Design review of the part built by this model. Coordinates are the model's own, in mm. Face numbers are marked on the shaded views. A direction names the side the tool comes from. Coordinates: 2 decimals unless noted, no trailing zeros. Write each loop counter-clockwise with the first axis right and the second up, starting at its lowest first coordinate (ties: lowest second). Pieces come first, ordered by that corner, then holes. Notation, with made-up numbers: (-19.5, 29.5) - (22.5, 29.5) arc R26 cw to (22.5, 52.5) - close; hole circle Ø3 at (89, 16). An arc over 180 degrees is marked (long way). Answer as a JSON object with one key per item and string values.
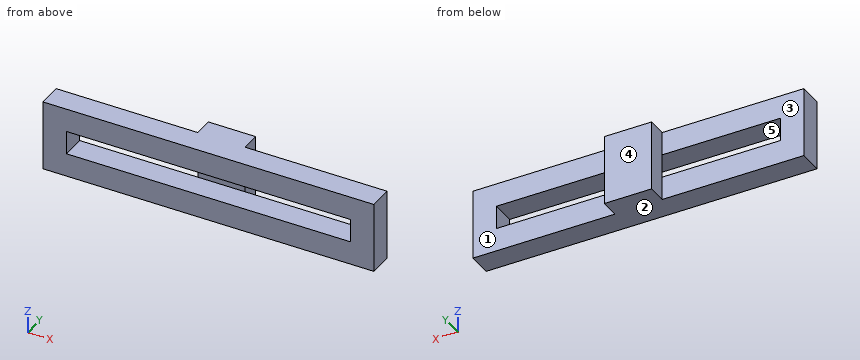
```python
from build123d import *

# Parameters (mm, degrees)
SKETCH2_W           = 70
SKETCH2_H           = 15
SKETCH2_W_2         = 60
SKETCH2_H_2         = 5
BOSS_EXTRUDE3_DEPTH = 5
SKETCH3_W           = 10
SKETCH3_H           = 15
BOSS_EXTRUDE4_DEPTH = 4


with BuildPart() as part:
    # Sketch2 → Boss-Extrude3 (new body)
    with BuildSketch(Plane(origin=(0, 0, 0), x_dir=(1, 0, 0), z_dir=(0, 1, 0))):
        Rectangle(SKETCH2_W, SKETCH2_H)
        Rectangle(SKETCH2_W_2, SKETCH2_H_2, mode=Mode.SUBTRACT)
    extrude(amount=BOSS_EXTRUDE3_DEPTH)

    # Sketch3 → Boss-Extrude4 (add)
    with BuildSketch(Plane(origin=(0, 5, 0), x_dir=(1, 0, 0), z_dir=(0, 1, 0))):
        Rectangle(SKETCH3_W, SKETCH3_H)
    extrude(amount=BOSS_EXTRUDE4_DEPTH)


solid = part.part
```
(1) Take a section at B-B, the plane y = 3.25. Write out the cut boundary in (x, z).
Solved:
{"outline": "(-35, -7.5) - (35, -7.5) - (35, 7.5) - (-35, 7.5) - close; hole (-30, -2.5) - (30, -2.5) - (30, 2.5) - (-30, 2.5) - close"}
(2) Take a section at D-D, the plane z = 6.75. Write out the cut boundary in (x, y).
Solved:
{"outline": "(-35, 0) - (35, 0) - (35, 5) - (5, 5) - (5, 9) - (-5, 9) - (-5, 5) - (-35, 5) - close"}
(3) Take a section at C-C, the plane x = 14. Write out the cut boundary in (y, z), and give its area (3 significant figures).
Solved:
{"outline": "(0, -7.5) - (5, -7.5) - (5, -2.5) - (0, -2.5) - close; (0, 2.5) - (5, 2.5) - (5, 7.5) - (0, 7.5) - close", "area": "50.0 mm^2"}
(4) For pin 1 (3 mm diameter, centred on y = 7, z = -3.5, fed in from +X); pin 2 (4.5 mm diameter, centred on x = 19.5, z = 2.5, fed in from +Y); pin 3 (4.5 mm diameter, centred on y = 7.5, z = 1.5, fed in from -X), all flat-tipped, find the tip position at first contact; note any pin that passes through.
Solved:
{"pin 1": "stops at x = 5", "pin 2": "stops at y = 5", "pin 3": "stops at x = -5"}
(5) The part is to be moulded in two halves that separate along X. For the marked faces 4 and 5, say which applies: pulls with the +X half, pulls with the -X half, needs draft (parallel to the pull), parting line crosses it, or undercut.
Solved:
{"face 4": "needs draft", "face 5": "undercut"}
(6) To check wall thickness, follow line 1 (Z direction, x = 19, y = 4); line 2 (X direction, y = 2.25, z = 0.5); line 3 (X direction, y = 5.75, z = -5.25). State the ranges of each line that lie inside material, in increasing order. Write a range as from..to.
Solved:
{"line 1": "z = -7.5..-2.5, 2.5..7.5", "line 2": "x = -35..-30, 30..35", "line 3": "x = -5..5"}
(7) Take a section at A-A, the plane z = -1.5. Write out the cut boundary in (x, y).
Solved:
{"outline": "(-35, 0) - (-30, 0) - (-30, 5) - (-35, 5) - close; (-5, 5) - (5, 5) - (5, 9) - (-5, 9) - close; (30, 0) - (35, 0) - (35, 5) - (30, 5) - close"}
(8) Tool access review of the marked faces 1, 2 and 3: name each direction out of +Z, -Z, +X, -X, +Y, -Y from which nothing blocks a thin tool from reaching the whole face with its end or side.
Solved:
{"face 1": "+Z, -Z, +X, +Y", "face 2": "-Z, +X, -X, +Y, -Y", "face 3": "+Z, -Z, -X, +Y"}
